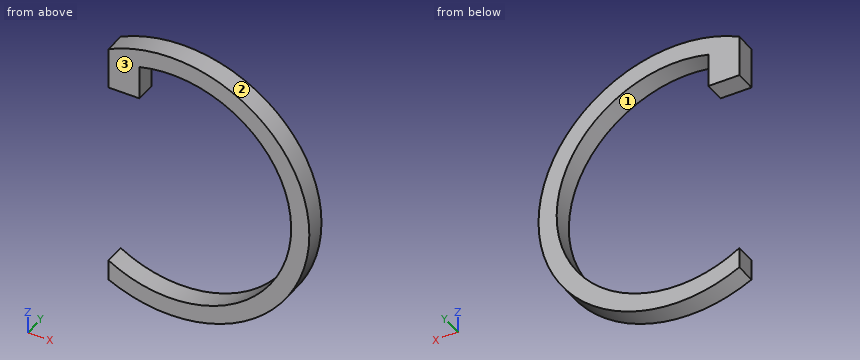
from build123d import *

# Parameters (mm, degrees)
BOSS_EXTRUDE1_DEPTH = 10
SKETCH2_W           = 20
SKETCH2_H           = 10
BOSS_EXTRUDE2_DEPTH = 15


with BuildPart() as part:
    # Sketch1 → Boss-Extrude1 (new body)
    with BuildSketch(Plane(origin=(0, 0, 0), x_dir=(1, 0, 0), z_dir=(0, 1, 0))):
        with BuildLine():
            Line((-20, 50), (-20, 60))
            ThreePointArc((-20, 60), (77.082039325, 0), (-20, -60))
            Line((-20, -60), (-20, -50))
            ThreePointArc((-20, -50), (68.309518948, 0), (-20, 50))
        make_face()
    extrude(amount=-BOSS_EXTRUDE1_DEPTH)

    # Sketch2 → Boss-Extrude2 (add)
    with BuildSketch(Plane.ZY.offset(20)):
        with Locations((50, -5)):
            Rectangle(SKETCH2_W, SKETCH2_H)
    extrude(amount=-BOSS_EXTRUDE2_DEPTH)


solid = part.part
The model under review builds one solid part; all positions refer to its coordinate system, in mm. Face numbers are marked on the shaded views. Round coordinates to 2 decimals unless told otherwise and drop trailing zeros. Loops run counter-clockwise (first coordinate to the right, second up) from the corner with the lowest first, then second, coordinate; pieces in that order, holes last. Notation, with made-up numbers: M 57.5,46 L 65.5,46 A19 ccw 65.5,56 Z; hole C -20,55.5 d6. An arc over 180 degrees is marked long. Answer as CSV lines item,"result". Start each with the question number.
Item 1: Consider section D-D (z = 0). Write out the cut boundary in (x, y), then the cut area to 3 significant figures.
Item 2: Mouldability with a two-part tool opening along Z and no side actions: class the marked faces 1, 2 and 3 as released by +Z, released by -Z, zero draft, split by the parting line, or undercut.
Item 3: Consider section C-C (y = -8). Write out the cut boundary in (x, z).
Item 4: Wall thickness on line 1 (Z direction, x = 10, y = -2); line 2 (Z direction, x = 34.5, y = -6); line 3 (X direction, y = -7.25, z = -18.5): over which ranges is each line inside the solid? List them lowest first. Write a range as [from, to].
Item 5: Consider section A-A (x = 10). Write out the cut boundary in (y, z).
Item 6: Consider section B-B (z = 53.5). Write out the cut boundary in (x, y), then the cut area to 3 significant figures.
Item 7: Insertion check: P1, Ø2, axis at x = 67, y = -8.5, coming from the +Z side; P2, Ø2, axis at y = -8, z = -46, coming from the -X side; P3, Ø3, axis at x = 38, z = 52, coming from the +Y side; P4, Ø1, axis at x = 37.5, z = 49.5, coming from the +Y side. Each pin has a flat end and moves straight along its axis. Give the tip position at first contact, or say it passes through.
Answer:
1,outline,"M 68.31,-10 L 77.08,-10 L 77.08,0 L 68.31,0 Z"
1,area,"87.7 mm^2"
2,face 1,"undercut"
2,face 2,"split by the parting line"
2,face 3,"zero draft"
3,outline,"M -20,-60 A67.08 ccw long -20,60 L -20,40 L -5,40 L -5,56.35 A58.31 cw long -20,-50 Z"
4,line 1,"z = [-67.08, -58.31], [58.31, 67.08]"
4,line 2,"z = [-62.45, -52.91], [52.91, 62.45]"
4,line 3,"x = [65.3, 74.48]"
5,outline,"M -10,-67.08 L 0,-67.08 L 0,-58.31 L -10,-58.31 Z; M -10,58.31 L 0,58.31 L 0,67.08 L -10,67.08 Z"
6,outline,"M -20,-10 L -5,-10 L -5,0 L -20,0 Z; M 33.19,-10 L 50.47,-10 L 50.47,0 L 33.19,0 Z"
6,area,"323 mm^2"
7,P1,"stops at z = 36.93"
7,P2,"stops at x = 44.51"
7,P3,"stops at y = 0"
7,P4,"passes through"
